Can you work these out from the model? Positions are in its coordinate system, mm. A direction names the side the tool comes from. Give positions to 0.01 mm unless a question says otherwise; leave off trailing zeros. Order: outer loops, then holes, each group sorted by start corner. A loop starts at its lowest first (then second) coordinate and runs counter-clockwise, first axis right, second up. Notation, with made-up numbers: M -24,-8.75 L -17,-8.75 A28 ccw -17,16.25 Z; hole C -19,85 d5. An arc over 180 degrees is marked long. Write each question's results on one line, items separated by ' | '.
from build123d import *

# Parameters (mm, degrees)
SKETCH_1_W      = 20.5
SKETCH_1_H      = 8.16
EXTRUDE_1_DEPTH = 0.23
SKETCH_2_W      = 12.82
SKETCH_2_H      = 3
EXTRUDE_2_DEPTH = 1.4
SKETCH_3_W      = 0.23
SKETCH_3_H      = 8.16
EXTRUDE_3_DEPTH = 12.27


with BuildPart() as part:
    # 草图1 → 凸台-拉伸1 (new body)
    with BuildSketch(Plane.XY):
        with Locations((-11.527217391, 1.472347826)):
            Rectangle(SKETCH_1_W, SKETCH_1_H)
    extrude(amount=EXTRUDE_1_DEPTH)

    # 草图2 → 凸台-拉伸2 (add)
    with BuildSketch(Plane.XY.offset(0.23)):
        with Locations((-15.367217391, 4.052347826)):
            Rectangle(SKETCH_2_W, SKETCH_2_H)
    extrude(amount=EXTRUDE_2_DEPTH)

    # 草图3 → 凸台-拉伸3 (add)
    with BuildSketch(Plane.XY.offset(0.23)):
        with Locations((-1.392217391, 1.472347826)):
            Rectangle(SKETCH_3_W, SKETCH_3_H)
    extrude(amount=EXTRUDE_3_DEPTH)


solid = part.part
(1) Imagine slicing it at C-C, the plane z = 7. Write out the boundary of the cut face in (x, y), plus the area to 3 significant figures.
Data:
outline: M -1.51,-2.61 L -1.28,-2.61 L -1.28,5.55 L -1.51,5.55 Z | area: 1.88 mm2
(2) Will these pins go through, and if not, where does the flat tip stop? P1, Ø0.9, axis at x = -12.5, y = 4, coming from the +Z side; P2, Ø1.5, axis at x = -11, z = 3, coming from the -Y side; P3, Ø0.7, axis at x = -17, z = 1, coming from the -Y side; P4, Ø2.5, axis at y = 2, z = 6.5, coming from the -X side.
Data:
P1: stops at z = 1.63 | P2: passes through | P3: stops at y = 2.55 | P4: stops at x = -1.51
(3) I need wall thicknesses on L1, parallel to Z at x = -7, y = 4.75; L2, parallel to X at y = 3, z = 3.75; L3, parallel to Z at x = -19.5, y = 4.5. Which ranges of each line are inside material? Lowest first, please. Write a range as from..to.
Data:
L1: z = 0..0.23 | L2: x = -1.51..-1.28 | L3: z = 0..1.63
(4) Imagine slicing it at D-D, the plane y = -0.25. Write out the boundary of the cut face in (x, z), plus the area to 3 significant figures.
Data:
outline: M -21.78,0 L -1.28,0 L -1.28,12.5 L -1.51,12.5 L -1.51,0.23 L -21.78,0.23 Z | area: 7.54 mm2
(5) For faces 4 (the face through (-15, 2.552, 1)), 5 (the face through (-14, 5.552, 1)), 6 (the face through (-15, 4, 1.63)), which set-ups out of +Z, -Z, +X, -X, +Y, -Y let a thin tool reach every point of the face, with its end or its side?
Data:
face 4: +Z, -X, -Y | face 5: +Z, -Z, +X, -X, +Y | face 6: +Z, -X, +Y, -Y
(6) Imagine slicing it at A-A, the plane x = -11. Write out the boundary of the cut face in (y, z).
Data:
outline: M -2.61,0 L 5.55,0 L 5.55,1.63 L 2.55,1.63 L 2.55,0.23 L -2.61,0.23 Z
(7) We'd pull the mould along X, two halves only. Please class faces 1 (the face through (-21.777, 3, 1)), 2 (the face through (-1.277, 1, 6)), 3 (the face through (-8.957, 4, 1)): +X half, -X half, draft (parallel to the pull), parting line (faces both ways), or undercut.
Data:
face 1: -X half | face 2: +X half | face 3: undercut
(8) Imagine slicing it at B-B, the plane y = 3.75. Write out the boundary of the cut face in (x, z), plus the area to 3 significant figures.
Data:
outline: M -21.78,0 L -1.28,0 L -1.28,12.5 L -1.51,12.5 L -1.51,0.23 L -8.96,0.23 L -8.96,1.63 L -21.78,1.63 Z | area: 25.5 mm2
